from build123d import *

# Parameters (mm, degrees)
SKETCH1_R                = 50
BOSS_EXTRUDE1_DEPTH      = 91
BOSS_EXTRUDE2_DEPTH      = 50
BOSS_EXTRUDE2_DEPTH_BACK = 50
SKETCH2_W                = 85
SKETCH2_H                = 77.5
SKETCH4_R                = 42.5
BOSS_EXTRUDE3_DEPTH      = 135
BOSS_EXTRUDE4_DEPTH      = 50
BOSS_EXTRUDE4_DEPTH_BACK = 50
SKETCH5_W                = 89
SKETCH5_H                = 60.5
SKETCH6_W                = 70
SKETCH6_H                = 45
BOSS_EXTRUDE5_DEPTH      = 58.5
SKETCH7_W                = 70.1
SKETCH7_H                = 45.1
BOSS_EXTRUDE6_DEPTH      = 70


with BuildPart() as part:
    # Sketch1 → Boss-Extrude1 (new body)
    with BuildSketch(Plane(origin=(0, 0, 0), x_dir=(1, 0, 0), z_dir=(0, 1, 0))):
        with Locations(Location((0, 0, 0), (0, 0, 270))):
            Circle(SKETCH1_R)
    extrude(amount=BOSS_EXTRUDE1_DEPTH)

    # Sketch2 → Boss-Extrude2 (add, two sides: drawn at the far end of the back side and taken through both)
    with BuildSketch(Plane(origin=(0, 0, 0), x_dir=(0, 0, -1), z_dir=(1, 0, 0)).offset(-BOSS_EXTRUDE2_DEPTH_BACK)):
        with Locations((0, 129.75)):
            Rectangle(SKETCH2_W, SKETCH2_H)
    extrude(amount=BOSS_EXTRUDE2_DEPTH + BOSS_EXTRUDE2_DEPTH_BACK)

    # Sketch4 → Boss-Extrude3 (add)
    with BuildSketch(Plane(origin=(0, 135.5, 0), x_dir=(1, 0, 0), z_dir=(0, 1, 0))):
        with Locations(Location((0, 0, 0), (0, 0, 270))):
            Circle(SKETCH4_R)
    extrude(amount=BOSS_EXTRUDE3_DEPTH)

    # Sketch5 → Boss-Extrude4 (add, two sides: drawn at the far end of the back side and taken through both)
    with BuildSketch(Plane(origin=(0, 0, 0), x_dir=(0, 0, -1), z_dir=(1, 0, 0)).offset(-BOSS_EXTRUDE4_DEPTH_BACK)):
        with Locations((-17, 300.75)):
            Rectangle(SKETCH5_W, SKETCH5_H)
    extrude(amount=BOSS_EXTRUDE4_DEPTH + BOSS_EXTRUDE4_DEPTH_BACK)

    # Sketch6 → Boss-Extrude5 (add)
    with BuildSketch(Plane.XY.offset(61.5)):
        with Locations((0, 300.75)):
            Rectangle(SKETCH6_W, SKETCH6_H)
    extrude(amount=BOSS_EXTRUDE5_DEPTH)

    # Sketch7 → Boss-Extrude6 (add)
    with BuildSketch(Plane.XY.offset(120)):
        with Locations((0, 300.75)):
            Rectangle(SKETCH7_W, SKETCH7_H)
    extrude(amount=BOSS_EXTRUDE6_DEPTH)


solid = part.part
Design review of the part built by this model. Coordinates are the model's own, in mm. A direction names the side the tool comes from. Give positions to 0.01 mm unless a question says otherwise; leave off trailing zeros. Loops run counter-clockwise (first coordinate to the right, second up) from the corner with the lowest first, then second, coordinate; pieces in that order, holes last. Notation, with made-up numbers: (57, -17) -> (104, -17) arc R22 cw to (104, 5) -> close; hole circle Ø8 at (-32, -22.75). An arc over 180 degrees is marked (long way). One line per question, with ' | ' between items. Start each with the question number.
(1) Draft analysis for pull direction Y (two halves, no side actions). For faces 1 (the face through (-25.861, 218.786, -33.727)), 2 (the face through (0, 91, 45)), 3 (the face through (-43, 91, -32)), 4 (the face through (-1, 300, -27.5)), state which applies: +Y half, -Y half, draft (parallel to the pull), parting line (faces both ways), or undercut.
(2) We need section A-A (y = 306.5). State the section outline as (x, z) points.
(3) For faces 5 (the face through (0, 323.3, 155)), 6 (the face through (42, 91, -32)), 7 (the face through (-35.05, 300, 155)), 8 (the face through (0, 91, -45)), list the 3-axis set-ups (+Z, -Z, +X, -X, +Y, -Y) from which the entire face can be reached by the end or side of a thin tool; tool diameter is ignored.
(4) We need section B-B (x = -5.5). State the section outline as (y, z) points, and give its area (3 significant figures).
(5) Insertion check: P1, Ø12, axis at x = 29, z = 50, coming from the -Y side; P2, Ø4, axis at x = -10.5, z = 33, coming from the -Y side; P3, Ø3, axis at x = -10, y = 228.5, coming from the -Z side; P4, Ø13.5, axis at y = 292.5, z = 159.5, coming from the +X side. Each pin has a flat end and moves straight along its axis. Give the tip position at first contact, or say it passes through.
(6) We need section D-D (x = 20.5). State the section outline as (y, z) points, and give its area (3 significant figures).
(7) For line 1 (Y direction, x = 31, z = 43.5); line 2 (Z direction, x = -36.5, y = 160.5); line 3 (Y direction, x = 42.5, z = -29.5), list the stretches that pass through material, from the lowest coordinate up.
(8) We need section C-C (z = 142.5). State the section outline as (x, y) points, and give its area (3 significant figures).
The answers:
1) face 1: undercut | face 2: undercut | face 3: -Y half | face 4: draft
2) outline: (-50, -27.5) -> (50, -27.5) -> (50, 61.5) -> (35, 61.5) -> (35, 120) -> (35.05, 120) -> (35.05, 190) -> (-35.05, 190) -> (-35.05, 120) -> (-35, 120) -> (-35, 61.5) -> (-50, 61.5) -> close
3) face 5: +Z, +X, -X, +Y | face 6: -Z, +X, -Y | face 7: +Z, -X, +Y, -Y | face 8: -Z, +X, -X, +Y
4) outline: (0, -49.7) -> (91, -49.7) -> (91, -42.5) -> (168.5, -42.5) -> (168.5, -42.14) -> (270.5, -42.14) -> (270.5, -27.5) -> (331, -27.5) -> (331, 61.5) -> (323.25, 61.5) -> (323.25, 120) -> (323.3, 120) -> (323.3, 190) -> (278.2, 190) -> (278.2, 120) -> (278.25, 120) -> (278.25, 61.5) -> (270.5, 61.5) -> (270.5, 42.14) -> (168.5, 42.14) -> (168.5, 42.5) -> (91, 42.5) -> (91, 49.7) -> (0, 49.7) -> close | area: 35,400 mm^2
5) P1: stops at y = 270.5 | P2: stops at y = 0 | P3: stops at z = -41.64 | P4: stops at x = 35.05
6) outline: (0, -45.6) -> (91, -45.6) -> (91, -42.5) -> (168.5, -42.5) -> (168.5, -37.23) -> (270.5, -37.23) -> (270.5, -27.5) -> (331, -27.5) -> (331, 61.5) -> (323.25, 61.5) -> (323.25, 120) -> (323.3, 120) -> (323.3, 190) -> (278.2, 190) -> (278.2, 120) -> (278.25, 120) -> (278.25, 61.5) -> (270.5, 61.5) -> (270.5, 37.23) -> (168.5, 37.23) -> (168.5, 42.5) -> (91, 42.5) -> (91, 45.6) -> (0, 45.6) -> close | area: 33,700 mm^2
7) line 1: y = 270.5 to 331 | line 2: z = -42.5 to 42.5 | line 3: y = 91 to 168.5
8) outline: (-35.05, 278.2) -> (35.05, 278.2) -> (35.05, 323.3) -> (-35.05, 323.3) -> close | area: 3,160 mm^2
